For this review, take the finished solid that the model builds, in its own axes (mm). Face numbers are marked on the shaded views. A direction names the side the tool comes from. Round coordinates to 2 decimals unless told otherwise and drop trailing zeros. Loops run counter-clockwise (first coordinate to the right, second up) from the corner with the lowest first, then second, coordinate; pieces in that order, holes last.
1. Draft analysis for pull direction X (two halves, no side actions). For the marked faces 1, 2 and 3, state which applies: released by +X, released by -X, zero draft, split by the parting line, or undercut.
2. To check wall thickness, follow line 1 along Y through (x, z) = (0, 13.25); line 2 along Y through (x, z) = (0, 23.3); line 3 along Y through (x, z) = (7.5, 22). State the ranges of each line that lie inside material, in increasing order.
3. Consider section A-A on x = -8.25. State the section outline as (y, z) points.
4. Tool access review of the marked faces 4, 5 and 6: name each direction out of +Z, -Z, +X, -X, +Y, -Y from which nothing blocks a thin tool from reaching the whole face with its end or side.
5. Consider section B-B on z = 7. State how many separate pieces and enclosed holes the cut face has, then the cut area to 3 significant figures.
6. Consider section C-C on z = -2.5. State the section outline as (x, y) points (1 decimal), then the cut area to 3 significant figures.
7. Clearance check with flat-ended pins moving along their axes: pin 1 Ø1.1 at (x, y) = (-8, -9.5) entering from +Z; pin 2 Ø2 at (x, z) = (10, 6.5) entering from +Y; pin 3 Ø2.5 at (x, y) = (5.2, -3) entering from -Z; pin 4 Ø1.6 at (x, y) = (-5.2, -3) entering from +Z. State where each tip first meets the part, or that it passes through.
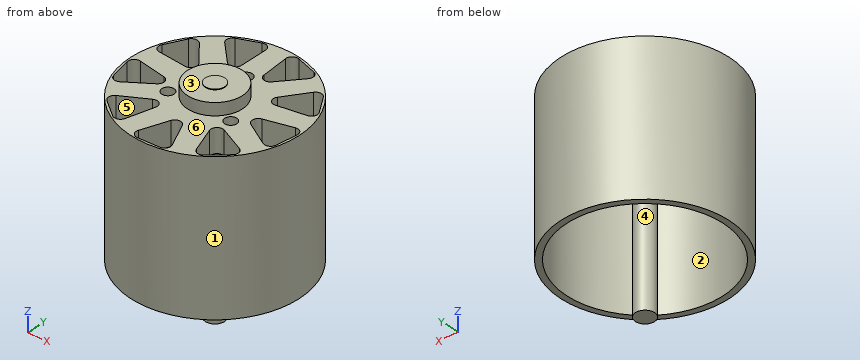
from build123d import *

# Parameters (mm, degrees)
SKETCH1_R                = 13.85
BOSS_EXTRUDE1_DEPTH      = 24.4
SKETCH2_R                = 12.85
CUT_EXTRUDE1_DEPTH       = 20.5
SKETCH3_R                = 1
CUT_EXTRUDE2_DEPTH       = 4.5
SKETCH4_R                = 4.5
BOSS_EXTRUDE2_DEPTH      = 2
BOSS_EXTRUDE3_DEPTH      = 0.1
BOSS_EXTRUDE3_DEPTH_BACK = 35
SKETCH5_R                = 1.5875


with BuildPart() as part:
    # Sketch1 → Boss-Extrude1 (new body)
    with BuildSketch(Plane.XY):
        Circle(SKETCH1_R)
    extrude(amount=BOSS_EXTRUDE1_DEPTH)

    # Sketch2 → Cut-Extrude1 (cut)
    with BuildSketch(Plane(origin=(0, 0, 0), x_dir=(-1, 0, 0), z_dir=(0, 0, -1))):
        Circle(SKETCH2_R)
    extrude(amount=-CUT_EXTRUDE1_DEPTH, mode=Mode.SUBTRACT)

    # Sketch3 → Cut-Extrude2 (cut)
    with BuildSketch(Plane.XY.offset(24.4)):
        with Locations((0, 6)):
            Circle(SKETCH3_R)
        with Locations((5.196152423, -3)):
            Circle(SKETCH3_R)
        with Locations((-5.196152423, -3)):
            Circle(SKETCH3_R)
        with BuildLine():
            Line((1.456483025, 7.691744175), (1.050821732, 12.328473971))
            ThreePointArc((1.050821732, 12.328473971), (1.421092958, 13.195514197), (2.347722229, 13.369346664))
            Line((2.347722229, 13.369346664), (5.745200753, 12.298125801))
            ThreePointArc((5.745200753, 12.298125801), (6.404544807, 11.624237864), (6.210539396, 10.70162124))
            Line((6.210539396, 10.70162124), (3.218722166, 7.136112308))
            ThreePointArc((3.218722166, 7.136112308), (2.151971923, 6.825182967), (1.456483025, 7.691744175))
        make_face()
        with BuildLine():
            Line((-2.121320344, 7.535533906), (-2.121320344, 12.189975257))
            ThreePointArc((-2.121320344, 12.189975257), (-2.565750111, 13.021444869), (-3.504003776, 13.113854789))
            Line((-3.504003776, 13.113854789), (-6.795190818, 11.75060048))
            ThreePointArc((-6.795190818, 11.75060048), (-7.393292666, 11.02181127), (-7.119614167, 10.119614167))
            Line((-7.119614167, 10.119614167), (-3.828427125, 6.828427125))
            ThreePointArc((-3.828427125, 6.828427125), (-2.738636911, 6.611654373), (-2.121320344, 7.535533906))
        make_face()
        with BuildLine():
            Line((6.05988858, 4.956008641), (8.729566463, 8.768703788))
            ThreePointArc((8.729566463, 8.768703788), (9.570533392, 9.194889379), (10.392109953, 8.73242696))
            Line((10.392109953, 8.73242696), (12.306161998, 5.727967071))
            ThreePointArc((12.306161998, 5.727967071), (12.378082031, 4.787920773), (11.63641873, 4.20585971))
            Line((11.63641873, 4.20585971), (7.052688802, 3.397624451))
            ThreePointArc((7.052688802, 3.397624451), (6.035649178, 3.845132596), (6.05988858, 4.956008641))
        make_face()
        with BuildLine():
            Line((7.82780492, -0.098698416), (12.323650028, 1.10595965))
            ThreePointArc((12.323650028, 1.10595965), (13.241814888, 0.891873631), (13.573913934, 0.009507632))
            Line((13.573913934, 0.009507632), (13.108933277, -3.52237111))
            ThreePointArc((13.108933277, -3.52237111), (12.559777106, -4.288717659), (11.617488416, -4.257870321))
            Line((11.617488416, -4.257870321), (7.586623965, -1.930649646))
            ThreePointArc((7.586623965, -1.930649646), (7.095179104, -0.93409805), (7.82780492, -0.098698416))
        make_face()
        with BuildLine():
            Line((5.933004342, -5.107223387), (10.151360783, -7.0742753))
            ThreePointArc((10.151360783, -7.0742753), (10.717104031, -7.828459701), (10.404332729, -8.717860424))
            Line((10.404332729, -8.717860424), (7.777888986, -11.124552702))
            ThreePointArc((7.777888986, -11.124552702), (6.864612886, -11.358617435), (6.162606158, -10.729295508))
            Line((6.162606158, -10.729295508), (4.57069346, -6.355551317))
            ThreePointArc((4.57069346, -6.355551317), (4.834795873, -5.276253837), (5.933004342, -5.107223387))
        make_face()
        with BuildLine():
            Line((1.262085094, -7.726021775), (3.229137007, -11.944378215))
            ThreePointArc((3.229137007, -11.944378215), (3.177741091, -12.885769735), (2.366448608, -13.366044698))
            Line((2.366448608, -13.366044698), (-1.192516003, -13.521432449))
            ThreePointArc((-1.192516003, -13.521432449), (-2.042579995, -13.113693876), (-2.175828011, -12.180364084))
            Line((-2.175828011, -12.180364084), (-0.583915313, -7.806619893))
            ThreePointArc((-0.583915313, -7.806619893), (0.31215792, -7.149591815), (1.262085094, -7.726021775))
        make_face()
        with BuildLine():
            Line((-3.999377796, -6.729728709), (-5.204035861, -11.225573817))
            ThreePointArc((-5.204035861, -11.225573817), (-5.848522222, -11.913684901), (-6.778723117, -11.760108112))
            Line((-6.778723117, -11.760108112), (-9.604929501, -9.59148368))
            ThreePointArc((-9.604929501, -9.59148368), (-9.994026995, -8.73272721), (-9.496168072, -7.932104935))
            Line((-9.496168072, -7.932104935), (-5.465303622, -5.60488426))
            ThreePointArc((-5.465303622, -5.60488426), (-4.356542193, -5.677556324), (-3.999377796, -6.729728709))
        make_face()
        with BuildLine():
            Line((-7.389487367, -2.584520788), (-11.202182514, -5.254198671))
            ThreePointArc((-11.202182514, -5.254198671), (-12.138196989, -5.367054496), (-12.752054958, -4.651486241))
            Line((-12.752054958, -4.651486241), (-13.523089739, -1.173573099))
            ThreePointArc((-13.523089739, -1.173573099), (-13.269157693, -0.265620429), (-12.373145554, 0.027674268))
            Line((-12.373145554, 0.027674268), (-7.789415626, -0.78056099))
            ThreePointArc((-7.789415626, -0.78056099), (-6.986767796, -1.54892913), (-7.389487367, -2.584520788))
        make_face()
        with BuildLine():
            Line((-7.321973674, 2.770013134), (-11.95870347, 3.175674427))
            ThreePointArc((-11.95870347, 3.175674427), (-12.748274483, 3.690880356), (-12.758558561, 4.633617738))
            Line((-12.758558561, 4.633617738), (-11.113645995, 7.793465378))
            ThreePointArc((-11.113645995, 7.793465378), (-10.335502037, 8.325773103), (-9.460590719, 7.974504374))
            Line((-9.460590719, 7.974504374), (-6.468773488, 4.408995442))
            ThreePointArc((-6.468773488, 4.408995442), (-6.347807098, 3.304459219), (-7.321973674, 2.770013134))
        make_face()
    extrude(amount=-CUT_EXTRUDE2_DEPTH, mode=Mode.SUBTRACT)

    # Sketch4 → Boss-Extrude2 (add)
    with BuildSketch(Plane.XY.offset(24.4)):
        Circle(SKETCH4_R)
    extrude(amount=BOSS_EXTRUDE2_DEPTH)

    # Sketch5 → Boss-Extrude3 (add, two sides: drawn at the far end of the back side and taken through both)
    with BuildSketch(Plane.XY.offset(26.4).offset(-BOSS_EXTRUDE3_DEPTH_BACK)):
        Circle(SKETCH5_R)
    extrude(amount=BOSS_EXTRUDE3_DEPTH + BOSS_EXTRUDE3_DEPTH_BACK)


solid = part.part
Resolved:
1. face 1: split by the parting line
1. face 2: undercut
1. face 3: zero draft
2. line 1: y = -13.85 to -12.85, -1.59 to 1.59, 12.85 to 13.85
2. line 2: y = -13.85 to -13.47, -7.21 to 5, 7 to 13.85
2. line 3: y = -11.64 to -11.3, -5.84 to -1.87, -0.25 to 3.48, 7.01 to 11.64
3. outline: (-11.12, 0) - (-9.85, 0) - (-9.85, 19.9) - (-10.63, 19.9) - (-10.63, 24.4) - (-11.12, 24.4) - close; (-7.21, 20.5) - (-3.19, 20.5) - (-3.19, 24.4) - (-7.21, 24.4) - close; (-0.7, 20.5) - (2.85, 20.5) - (2.85, 24.4) - (-0.7, 24.4) - close; (6.53, 20.5) - (9.85, 20.5) - (9.85, 0) - (11.12, 0) - (11.12, 24.4) - (6.53, 24.4) - close
4. face 4: -Z
4. face 5: +Z, -Z
4. face 6: +Z
5. separate pieces: 2
5. enclosed holes: 1
5. area: 91.8 mm2
6. outline: circle Ø3.2 at (0, 0)
6. area: 7.92 mm2
7. pin 1: stops at z = 19.9
7. pin 2: stops at y = 10.53
7. pin 3: stops at z = 20.5
7. pin 4: passes through
